```python
from build123d import *

# Parameters (mm, degrees)
F0_W     = 76.2
F0_H     = 50.8
F1_DEPTH = 495.3
F2_W     = 25.4
F2_H     = 444.5
F3_DEPTH = 50.8
F4_R     = 6.35
F5_DEPTH = 76.2


with BuildPart() as f1:
    # F0 (on Front) → F1 (new body)
    with BuildSketch(Plane.XZ):
        with Locations((38.1, -25.4)):
            Rectangle(F0_W, F0_H)
    extrude(amount=F1_DEPTH)

    # F2 (on face) → F3 (cut)
    with BuildSketch(Plane.XY):
        with Locations((38.1, -247.65)):
            Rectangle(F2_W, F2_H)
    extrude(amount=-F3_DEPTH, mode=Mode.SUBTRACT)

    # F4 (on face) → F5 (cut)
    with BuildSketch(Plane.YZ.offset(76.2)):
        with Locations((-450.85, -12.7)):
            Circle(F4_R)
        with Locations((-400.05, -12.7)):
            Circle(F4_R)
        with Locations((-349.25, -12.7)):
            Circle(F4_R)
        with Locations((-298.45, -12.7)):
            Circle(F4_R)
        with Locations((-247.65, -12.7)):
            Circle(F4_R)
        with Locations((-196.85, -12.7)):
            Circle(F4_R)
        with Locations((-146.05, -12.7)):
            Circle(F4_R)
        with Locations((-95.25, -12.7)):
            Circle(F4_R)
        with Locations((-44.45, -12.7)):
            Circle(F4_R)
        with Locations((-69.85, -38.1)):
            Circle(F4_R)
        with Locations((-120.65, -38.1)):
            Circle(F4_R)
        with Locations((-171.45, -38.1)):
            Circle(F4_R)
        with Locations((-222.25, -38.1)):
            Circle(F4_R)
        with Locations((-273.05, -38.1)):
            Circle(F4_R)
        with Locations((-323.85, -38.1)):
            Circle(F4_R)
        with Locations((-374.65, -38.1)):
            Circle(F4_R)
        with Locations((-425.45, -38.1)):
            Circle(F4_R)
    extrude(amount=-F5_DEPTH, mode=Mode.SUBTRACT)


solid = f1.part
```
Model file for the job. Use its own axes, mm. A direction names the side the tool comes from. Give positions to 0.01 mm unless a question says otherwise; leave off trailing zeros. Write each loop counter-clockwise with the first axis right and the second up, starting at its lowest first coordinate (ties: lowest second). Pieces come first, ordered by that corner, then holes. Notation, with made-up numbers: (-12.5, 42.25) - (-3.5, 42.25) arc R29 ccw to (-3.5, 70.25) - close; hole circle Ø6 at (55.5, 34.25). An arc over 180 degrees is marked (long way). One line per question, with ' | ' between items. Start each with the question number.
(1) 3-axis set-ups, long thin cutter, end or side, ignore diameter. For faces 1 (the face through (38, -25.4, -25)), 2 (the face through (12.878, -114.593, -36.193)): which of +Z, -Z, +X, -X, +Y, -Y reach the whole face in a straight line?
(2) Pin check, flat tip, straight feed: P1, Ø5, axis at y = -347, z = -14.5, coming from the +X side. Stop position of the tip, or through.
(3) Slice it at C-C on x = 67.5. Give the number of separate pieces and of enclosed holes in the cut face, plus the area to 3 significant figures.
(4) Wall check: line 1 along Z through (x, y) = (10, -273.05); line 2 along Z through (x, y) = (68, -298.45); line 3 along Y through (x, z) = (34.5, -27). Give the ranges that are in metal, low to high. Write a range as from..to.
(5) Slice it at A-A on y = -171.45. Write the cut outline in (x, z).
(6) Slice it at D-D on y = -399. Write the cut outline in (x, z).
(7) Slice it at B-B on x = 38. Write the cut outline in (y, z), plus the area to 3 significant figures.
(8) Two-plate mould, pull along Z, no slides. Class faces 3 (the face through (63.678, -330.194, -37.821)), 4 (the face through (38, -469.9, -25)), 5 (the face through (21, -244, 0)), 6 (the face through (21, -244, -50.8)): +Z half, -Z half, draft (parallel to the pull), parting line (faces both ways), or undercut.
Results below:
1) face 1: +Z, -Z | face 2: +X, -X
2) P1: through
3) separate pieces: 1 | enclosed holes: 17 | area: 23,000 mm^2
4) line 1: -50.8..-44.45, -31.75..0 | line 2: -50.8..-19.05, -6.35..0 | line 3: -495.3..-469.9, -25.4..0
5) outline: (0, -50.8) - (25.4, -50.8) - (25.4, -44.45) - (0, -44.45) - close; (0, -31.75) - (25.4, -31.75) - (25.4, 0) - (0, 0) - close; (50.8, -50.8) - (76.2, -50.8) - (76.2, -44.45) - (50.8, -44.45) - close; (50.8, -31.75) - (76.2, -31.75) - (76.2, 0) - (50.8, 0) - close
6) outline: (0, -50.8) - (25.4, -50.8) - (25.4, -18.96) - (0, -18.96) - close; (0, -6.44) - (25.4, -6.44) - (25.4, 0) - (0, 0) - close; (50.8, -50.8) - (76.2, -50.8) - (76.2, -18.96) - (50.8, -18.96) - close; (50.8, -6.44) - (76.2, -6.44) - (76.2, 0) - (50.8, 0) - close
7) outline: (-495.3, -50.8) - (-469.9, -50.8) - (-469.9, 0) - (-495.3, 0) - close; (-25.4, -50.8) - (0, -50.8) - (0, 0) - (-25.4, 0) - close | area: 2,580 mm^2
8) face 3: undercut | face 4: draft | face 5: +Z half | face 6: -Z half
